Autodesk Inventor part; units mm, degrees
ref_plane "Work Plane1" through (0, 50.8, 678.442) normal (0.866, 0, 0.5) x (0, -1, 0)
ref_plane "Work Plane2" through (0, 0, 678.442) normal (-0.866, 0, 0.5) x (0, 1, 0)
ref_plane "Work Plane3" through (0, 0, -678.442) normal (0.866, 0, 0.5) x (0, 1, 0)
sketch "Sketch1" plane through (0, 0, 0) normal (0, 1, 0) x (-1, 0, 0)
  line L0 (-100.4, 678.442) -> (100.4, 678.442)
  line L1 (100.4, 678.442) -> (100.4, -678.442)
  line L2 (100.4, -678.442) -> (-100.4, -678.442)
  line L3 (-100.4, -678.442) -> (-100.4, 678.442)
  line L4 (-100.4, 678.442) -> (100.4, -678.442) construction
  line L5 (100.4, 678.442) -> (-100.4, -678.442) construction
  point P0 (0, 0)
  dimension "d0" = 200.8
  dimension "d1" = 1356.884
extrude "Extrusion1" add sketch "Sketch1" along normal blind 50.8
sketch "Sketch2" plane through (0, 50.8, 0) normal (0, 1, 0) x (1, 0, 0)
  line L0 (-100.4, -678.442) -> (100.4, -678.442)
  line L1 (0, -678.442) -> (-100.4, -504.5441)
  line L2 (0, -678.442) -> (200.8, -678.442) construction
  line L3 (-100.4, -504.5441) -> (100.4, -504.5441)
  line L4 (100.4, -678.442) -> (100.4, 678.442)
  line L5 (0, -678.442) -> (100.4, -504.5441)
  line L6 (0, 678.442) -> (-100.4062, 504.5334)
  line L7 (0, 678.442) -> (200.8124, 678.442) construction
  line L8 (-100.4062, 504.5334) -> (100.4, 504.5334)
  line L9 (0, 678.442) -> (100.4, 504.5334)
  point P0 (0, 0)
  dimension "d10" = 150
  dimension "d11" = 150
  dimension "d12" = 60
  dimension "d4" = 200.8
  dimension "d5" = 120
  dimension "d6" = 200.8124
  dimension "d7" = 120
ref_plane "Work Plane1" through (0, 50.8, 678.442) normal (0.866, 0, 0.5) x (0, -1, 0)
split "Split1" plane through (0, 50.8, 678.442) removes the side toward (0.866, 0, 0.5)
ref_plane "Work Plane2" through (0, 0, 678.442) normal (-0.866, 0, 0.5) x (0, 1, 0)
ref_plane "Work Plane3" through (0, 0, -678.442) normal (0.866, 0, 0.5) x (0, 1, 0)
split "Split2" plane through (0, 0, -678.442) removes the side toward (-0.866, 0, -0.5)
split "Split3" plane through (0, 0, 678.442) removes the side toward (-0.866, 0, 0.5)
ref_plane "Work Plane4" through (0, 0, -678.442) normal (0.866, 0, -0.5) x (0, 1, 0)
split "Split4" plane through (0, 0, -678.442) removes the side toward (0.866, 0, -0.5)
sketch "Sketch3" plane through (0, 50.8, 0) normal (0, 1, 0) x (1, 0, 0)
  line L0 (-75, -519.2088) -> (75, -519.2088)
  line L1 (75, -519.2088) -> (0, -649.1126)
  line L2 (0, -649.1126) -> (-75, -519.2088)
  line L3 (-75.0016, 519.2007) -> (74.9984, 519.2007)
  line L4 (74.9984, 519.2007) -> (-0.0016, 649.1046)
  line L5 (-0.0016, 649.1046) -> (-75.0016, 519.2007)
  circle A0 centre (-0.0016, 562.502) radius 43.3013
  circle A1 centre (-0.0016, 562.502) radius 57.9687
  point P0 (0, 0)
  dimension "d6" = 200.8124
  dimension "d7" = 120
  dimension "d8" = 150
  dimension "d9" = 150
  dimension "d10" = 150
  dimension "d11" = 150
  dimension "d12" = 60
sketch "Sketch4" plane through (0, 50.8, 0) normal (0, 1, 0) x (1, 0, 0)
  point P0 (0, 0)
sketch "Sketch5" plane through (0, 50.8, 0) normal (0, 1, 0) x (1, 0, 0)
  point P0 (0, 0)
extrude "Extrusion2" cut sketch "Sketch3" against normal blind 25.4 contours L0 L1 L2
sketch "Sketch6" plane through (0, 50.8, 0) normal (0, 1, 0) x (1, 0, 0)
  line L0 (-75.0016, 519.2007) -> (74.9984, 519.2007)
  line L1 (74.9984, 519.2007) -> (-0.0016, 649.1046)
  line L2 (-0.0016, 649.1046) -> (-75.0016, 519.2007)
  point P0 (0, 0)
  dimension "d15" = 150
  dimension "d16" = 150
extrude "Extrusion3" cut sketch "Sketch6" against normal blind 25.4
sketch "Sketch11" plane through (0, 50.8, 0) normal (0, 1, 0) x (1, 0, 0)
  line L0 (-20, 295) -> (20, 295)
  line L1 (20, 295) -> (20, 305)
  line L2 (20, 305) -> (-20, 305)
  line L3 (-20, 305) -> (-20, 295)
  line L4 (-20, 295) -> (20, 305) construction
  line L5 (20, 295) -> (-20, 305) construction
  point P0 (0, 0)
  point P1 (0, 300)
  dimension "d42" = 40
  dimension "d43" = 10
extrude "Extrusion6" cut sketch "Sketch11" against normal blind 50.8
sketch "Sketch12" plane through (0, 50.8, 0) normal (0, 1, 0) x (1, 0, 0)
  line L0 (-20, -305) -> (20, -305)
  line L1 (20, -305) -> (20, -295)
  line L2 (20, -295) -> (-20, -295)
  line L3 (-20, -295) -> (-20, -305)
  line L4 (-20, -305) -> (20, -295) construction
  line L5 (20, -305) -> (-20, -295) construction
  point P0 (0, 0)
  point P1 (0, -300)
  dimension "d46" = 40
  dimension "d47" = 10
extrude "Extrusion7" cut sketch "Sketch12" against normal blind 50.8
sketch "Sketch13" plane through (0, 50.8, 0) normal (0, 1, 0) x (1, 0, 0)
  circle A0 centre (0, -40) radius 2.5
  circle A1 centre (0, -120) radius 2.5
  circle A2 centre (0, -200) radius 2.5
  circle A3 centre (0, -280) radius 2.5
  circle A4 centre (0, 40) radius 2.5
  circle A5 centre (0, 100) radius 2.5
  circle A6 centre (0, 200) radius 2.5
  point P0 (0, 0)
  dimension "d50" = 5
  dimension "d51" = 5
  dimension "d52" = 5
  dimension "d53" = 5
  dimension "d54" = 5
  dimension "d55" = 5
  dimension "d56" = 5
extrude "Extrusion8" cut sketch "Sketch13" against normal blind 50.8 contours A3
sketch "Sketch14" plane through (0, 50.8, 0) normal (0, 1, 0) x (1, 0, 0)
  circle A0 centre (0, -200) radius 2.5
  point P0 (0, 0)
  dimension "d59" = 5
extrude "Extrusion9" cut sketch "Sketch14" against normal blind 50.8
sketch "Sketch15" plane through (0, 50.8, 0) normal (0, 1, 0) x (1, 0, 0)
  circle A0 centre (0, -120) radius 2.5
  point P0 (0, 0)
  dimension "d62" = 5
extrude "Extrusion10" cut sketch "Sketch15" against normal blind 50.8
sketch "Sketch16" plane through (0, 50.8, 0) normal (0, 1, 0) x (1, 0, 0)
  circle A0 centre (0, -40) radius 2.5
  circle A1 centre (0, 40) radius 2.5
  point P0 (0, 0)
  dimension "d65" = 5
  dimension "d66" = 5
extrude "Extrusion11" cut sketch "Sketch16" against normal blind 50.8
sketch "Sketch17" plane through (0, 50.8, 0) normal (0, 1, 0) x (1, 0, 0)
  circle A0 centre (0, 120) radius 2.5
  circle A1 centre (0, 200) radius 2.5
  circle A2 centre (0, 280) radius 2.5
  point P0 (0, 0)
  dimension "d69" = 5
  dimension "d70" = 5
  dimension "d71" = 5
extrude "Extrusion12" cut sketch "Sketch17" against normal blind 50.8
sketch "Sketch18" plane through (0, 0, 0) normal (0, -1, 0) x (1, 0, 0)
  circle A0 centre (-10, -240) radius 2.5
  circle A1 centre (-10, -160) radius 2.5
  circle A2 centre (-10, 0) radius 2.5
  circle A3 centre (-10, 80) radius 2.5
  circle A4 centre (-10, 160) radius 2.5
  point P0 (0, 0)
  dimension "d74" = 5
  dimension "d75" = 5
  dimension "d76" = 5
  dimension "d77" = 5
  dimension "d78" = 5
extrude "Extrusion13" cut sketch "Sketch18" against normal blind 50.8
sketch "Sketch19" plane through (0, 0, 0) normal (0, -1, 0) x (1, 0, 0)
  line L0 (74.9984, -519.2007) -> (-75.0016, -519.2007)
  line L1 (75.0016, 519.2007) -> (-75.0016, 519.2007)
  line L2 (-75.0016, 519.2007) -> (-75.0016, -519.2007)
  line L3 (-75.0016, -519.2007) -> (75.0016, -519.2007)
  line L4 (75.0016, -519.2007) -> (75.0016, 519.2007)
  line L5 (75.0016, 519.2007) -> (-75.0016, -519.2007) construction
  line L6 (-75.0016, 519.2007) -> (75.0016, -519.2007) construction
  point P0 (0, 0)
extrude "Extrusion14" cut sketch "Sketch19" against normal blind 25.4
properties part number "top"
Input: part model. Units: mm. Frame: model coordinates. A direction names the side the tool comes from. Give positions to 0.01 mm unless a question says otherwise; leave off trailing zeros. Write each loop counter-clockwise with the first axis right and the second up, starting at its lowest first coordinate (ties: lowest second). Pieces come first, ordered by that corner, then holes. Notation, with made-up numbers: (-18, 13.5) - (2, 13.5) arc R16 cw to (2, 31.5) - close; hole circle Ø3 at (-18, 75.25). An arc over 180 degrees is marked (long way). Write item = value, one per line. Start each with the question number.
1. First-contact query: pin 1 Ø4 at (x, z) = (51, 382) entering from -Y; pin 2 Ø4 at (x, y) = (-26.5, 31) entering from -Z; pin 3 Ø20.5 at (x, y) = (31, 16) entering from -Z. Flat tips, straight axial feed; report the tip coordinate or a pass-through.
2. Ray query, L1, parallel to X at y = 12.5, z = -479.5; L2, parallel to Z at x = 52, y = 44; L3, parallel to Z at x = 37, y = 30.5. Return the intervals inside material, ascending.
3. Section query A-A, the plane y = 34. Count the separate pieces of the cut face and the enclosed holes in it, then the cut area to 3 significant figures.
4. Mould query, pull axis X, two halves, no side actions, for faces 4 (the flat face through (-50.9, 25.76, -590.28)), 5 (the flat face through (49.497, 25.044, 592.71)), 6 (the flat face through (1, 13, 519.201)). Classes: released by +X, released by -X, zero draft, split by the parting line, or undercut.
5. Access query for faces 1 (the flat face through (-1, 25.4, 7)), 2 (the flat face through (0, 38, -305)), 3 (the flat face through (-1, 38, 519.209)). Directions: +Z, -Z, +X, -X, +Y, -Y. A direction counts if a zero-diameter tool reaches every point of the face in a straight line with its end or side. Return the directions, or none.
6. Section query C-C, the plane z = -225.5. Output: boundary loops of the cut face in (x, y), then the cut area to 3 significant figures.
Check sheet entries:
q1.pin_1 = 25.4
q1.pin_2 = -636.01
q1.pin_3 = -642.5
q2.L1 = -100.4 to -75, 75 to 100.4
q2.L2 = -588.38 to -559.04, -519.2 to 519.21, 559.05 to 588.38
q2.L3 = -614.36 to -585.02, -519.2 to 519.21, 585.03 to 614.36
q3.separate_pieces = 1
q3.enclosed_holes = 17
q3.area = 217,000 mm2
q4.face_4 = released by -X
q4.face_5 = released by +X
q4.face_6 = undercut
q5.face_1 = -Y
q5.face_2 = +Y, -Y
q5.face_3 = +Y
q6.outline = (-100.4, 0) - (-75, 0) - (-75, 25.4) - (75, 25.4) - (75, 0) - (100.4, 0) - (100.4, 50.8) - (-100.4, 50.8) - close
q6.area = 6,390 mm2
